```python
from build123d import *

# Parameters (mm, degrees)
F0_R     = 5.150035
F0_R_2   = 3.961987
F1_DEPTH = 9
F0_R_3   = 7.741214
F2_DEPTH = 6
F3_DEPTH = 7


with BuildPart() as f1:
    # F0 (on Top) → F1 (new body)
    with BuildSketch(Plane.XY):
        with BuildLine():
            add(Edge.make_bspline(
                [(-91.317542, -10.967116), (-86.64373, -13.858178), (-75.341257, -14.445624), (-67.806959, -14.301113)],
                knots=[1.221144, 1.221144, 1.221144, 1.221144, 24.488166, 24.488166, 24.488166, 24.488166], degree=3))
            add(Edge.make_bspline(
                [(-40.39795, -14.383757), (-39.723586, -5.585385), (-61.1616, 5.31907), (-67.806959, -14.301113)],
                knots=[0, 0, 0, 0, 27.409134, 27.409134, 27.409134, 27.409134], degree=3))
            add(Edge.make_bspline(
                [(-40.39795, -14.383757), (-33.312143, -14.897632), (-19.552754, -13.304103), (-16.391562, -11.32243)],
                knots=[0, 0, 0, 0, 21.643832, 21.643832, 21.643832, 21.643832], degree=3))
            Line((-16.391562, -11.32243), (-15.747862, -10.386982))
            ThreePointArc((-15.747862, -10.386982), (-25.2145, 12.283506), (-46.526868, 24.50444))
            Line((-46.526868, 24.50444), (-46.526868, 23.27941))
            Line((-46.526868, 23.27941), (-59.356738, 23.27941))
            Line((-59.356738, 23.27941), (-59.356738, 24.820338))
            ThreePointArc((-59.356738, 24.820338), (-81.928546, 12.942305), (-91.997162, -10.49265))
            Line((-91.997162, -10.49265), (-91.317542, -10.967116))
        make_face()
        with BuildLine():
            add(Edge.make_bspline(
                [(-67.806959, -20.841723), (-61.319683, -39.555024), (-41.559912, -31.048808), (-40.048894, -20.841723)],
                knots=[0, 0, 0, 0, 27.758066, 27.758066, 27.758066, 27.758066], degree=3))
            add(Edge.make_bspline(
                [(-91.241727, -17.905849), (-86.307066, -19.370394), (-73.921331, -20.639642), (-67.806959, -20.841723)],
                knots=[1.260164, 1.260164, 1.260164, 1.260164, 24.380885, 24.380885, 24.380885, 24.380885], degree=3))
            add(Edge.make_bspline(
                [(-91.979973, -17.664781), (-91.757507, -17.745623), (-91.510684, -17.826026), (-91.241727, -17.905849)],
                knots=[0, 0, 0, 0, 1.260164, 1.260164, 1.260164, 1.260164], degree=3))
            ThreePointArc((-91.979973, -17.664781), (-53.883548, -51.259255), (-16.087698, -17.32697))
            add(Edge.make_bspline(
                [(-16.761014, -17.670424), (-16.49914, -17.558172), (-16.273367, -17.443651), (-16.087698, -17.32697)],
                knots=[22.749196, 22.749196, 22.749196, 22.749196, 24.217605, 24.217605, 24.217605, 24.217605], degree=3))
            add(Edge.make_bspline(
                [(-40.048894, -20.841723), (-33.540111, -20.603637), (-20.818081, -19.409468), (-16.761014, -17.670424)],
                knots=[0, 0, 0, 0, 22.749196, 22.749196, 22.749196, 22.749196], degree=3))
        make_face()
        with Locations((-53.800639, -17.735399)):
            Circle(F0_R)
        with BuildLine():
            Line((-59.356738, 35.656463), (-59.356738, 24.820338))
            ThreePointArc((-59.356738, 24.820338), (-52.928445, 25.204892), (-46.526868, 24.50444))
            Line((-46.526868, 24.50444), (-46.526868, 35.656463))
            Line((-46.526868, 35.656463), (-59.356738, 35.656463))
        make_face()
        with Locations((-53.168215, 29.618876)):
            Circle(F0_R_2, mode=Mode.SUBTRACT)
        with BuildLine():
            ThreePointArc((-46.526868, 24.50444), (-52.928445, 25.204892), (-59.356738, 24.820338))
            Line((-59.356738, 24.820338), (-59.356738, 23.27941))
            Line((-59.356738, 23.27941), (-46.526868, 23.27941))
            Line((-46.526868, 23.27941), (-46.526868, 24.50444))
        make_face()
    extrude(amount=F1_DEPTH)

    # F0 (on Top) → F2 (join)
    with BuildSketch(Plane.XY):
        with BuildLine():
            add(Edge.make_bspline(
                [(-91.241727, -17.905849), (-86.307066, -19.370394), (-73.921331, -20.639642), (-67.806959, -20.841723)],
                knots=[1.260164, 1.260164, 1.260164, 1.260164, 24.380885, 24.380885, 24.380885, 24.380885], degree=3))
            Line((-67.806959, -20.841723), (-67.806959, -14.301113))
            add(Edge.make_bspline(
                [(-91.317542, -10.967116), (-86.64373, -13.858178), (-75.341257, -14.445624), (-67.806959, -14.301113)],
                knots=[1.221144, 1.221144, 1.221144, 1.221144, 24.488166, 24.488166, 24.488166, 24.488166], degree=3))
            ThreePointArc((-91.317542, -10.967116), (-91.519995, -14.439109), (-91.241727, -17.905849))
        make_face()
        with BuildLine():
            Line((-40.39795, -14.383757), (-40.048894, -20.841723))
            add(Edge.make_bspline(
                [(-40.048894, -20.841723), (-33.540111, -20.603637), (-20.818081, -19.409468), (-16.761014, -17.670424)],
                knots=[0, 0, 0, 0, 22.749196, 22.749196, 22.749196, 22.749196], degree=3))
            ThreePointArc((-16.761014, -17.670424), (-16.375445, -14.508116), (-16.391562, -11.32243))
            add(Edge.make_bspline(
                [(-40.39795, -14.383757), (-33.312143, -14.897632), (-19.552754, -13.304103), (-16.391562, -11.32243)],
                knots=[0, 0, 0, 0, 21.643832, 21.643832, 21.643832, 21.643832], degree=3))
        make_face()
        with BuildLine():
            Line((-67.806959, -14.301113), (-67.806959, -20.841723))
            add(Edge.make_bspline(
                [(-67.806959, -20.841723), (-61.319683, -39.555024), (-41.559912, -31.048808), (-40.048894, -20.841723)],
                knots=[0, 0, 0, 0, 27.758066, 27.758066, 27.758066, 27.758066], degree=3))
            Line((-40.048894, -20.841723), (-40.39795, -14.383757))
            add(Edge.make_bspline(
                [(-40.39795, -14.383757), (-39.723586, -5.585385), (-61.1616, 5.31907), (-67.806959, -14.301113)],
                knots=[0, 0, 0, 0, 27.409134, 27.409134, 27.409134, 27.409134], degree=3))
        make_face()
        with Locations((-53.800639, -17.735399)):
            Circle(F0_R_3, mode=Mode.SUBTRACT)
    extrude(amount=F2_DEPTH)

    # F0 (on Top) → F3 (join)
    with BuildSketch(Plane.XY):
        with Locations((-53.800639, -17.735399)):
            Circle(F0_R_3)
        with Locations((-53.800639, -17.735399)):
            Circle(F0_R, mode=Mode.SUBTRACT)
    extrude(amount=F3_DEPTH)


solid = f1.part
```
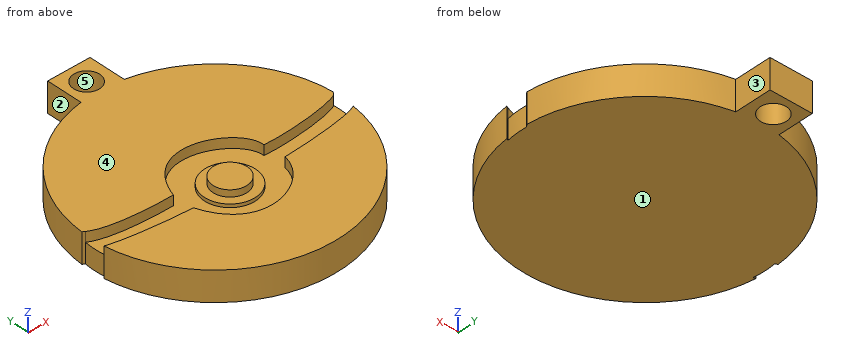
Could you check a few things on this model? Use its own coordinates, in mm. Face numbers are marked on the shaded views. A direction names the side the tool comes from. Give positions to 0.01 mm unless a question says otherwise; leave off trailing zeros. Loops run counter-clockwise (first coordinate to the right, second up) from the corner with the lowest first, then second, coordinate; pieces in that order, holes last. Notation, with made-up numbers: (66, 36) - (117, 36) arc R11 cw to (117, 47) - close; hole circle Ø8 at (-5.5, 45). An arc over 180 degrees is marked (long way). Answer in a Markdown table with one row per item. Add a question column.
Q1. If we section it at B-B (y = 16.5): List the corners of the cut face in (x, z) for me.
Q2. If we section it at A-A (y = -39.5): List the corners of the cut face in (x, z) for me.
Q3. We'd pull the mould along X, two halves only. Please class the marked faces 3, 4 and 5: +X half, -X half, draft (parallel to the pull), parting line (faces both ways), or undercut.
Q4. Please list where these lines run through material, in increasing order: L1, parallel to Y at x = -60, z = 6.5; L2, parallel to Z at x = -20, y = -13; L3, parallel to Y at x = -83, z = 8.25. Write a range as from..to.
Q5. For pin 1 (4.5 mm diameter, centred on y = 29.5, z = 3.5, fed in from -X); pin 2 (1 mm diameter, centred on x = -46, y = -12, fed in from -Z); pin 3 (3 mm diameter, centred on y = -21, z = 5, fed in from -X); pin 4 (1.5 mm diameter, centred on x = -32.5, z = 5.5, fed in from -Y), each with a flat end and sliding along its axis, tell me the tip position at first contact or that it passes through.
Q6. Which directions (+Z, -Z, +X, -X, +Y, -Y) give clear straight access to the entire face, cutting with the end or side of a thin tool? Please do the marked faces 1 and 2.
The answers:
| question | item | result |
|---|---|---|
| 1 | outline | (-78.16, 0) - (-29.58, 0) - (-29.58, 9) - (-78.16, 9) - close |
| 2 | outline | (-81.63, 0) - (-26.48, 0) - (-26.48, 9) - (-81.63, 9) - close |
| 3 | face 3 | +X half |
| 3 | face 4 | draft |
| 3 | face 5 | undercut |
| 4 | L1 | y = -50.79..-30.68, -22.37..-13.1, -4.48..24.72 |
| 4 | L2 | z = 0..6 |
| 4 | L3 | y = -37.99..-19.46, -13.46..11.73 |
| 5 | pin 1 | stops at x = -59.36 |
| 5 | pin 2 | stops at z = 0 |
| 5 | pin 3 | stops at x = -91.71 |
| 5 | pin 4 | stops at y = -45.1 |
| 6 | face 1 | -Z, +X, -X, +Y, -Y |
| 6 | face 2 | +Z, -Z, -X, +Y |
